Part model, mm, in its own coordinate system. Coordinates: 2 decimals unless noted, no trailing zeros. Write each loop counter-clockwise with the first axis right and the second up, starting at its lowest first coordinate (ties: lowest second). Pieces come first, ordered by that corner, then holes. Notation, with made-up numbers: M 50,-34 L 75,-34 A28 ccw 75,-4 Z; hole C 32,50.5 d3. An arc over 180 degrees is marked long. Use a Markdown table: item, result. Add a question column.
Q1. Mould opens along X. For faces 1 (the cylindrical face through (326.824, -3.131, 319.715)), 2 (the flat face through (276, -6.35, 283)), 3 (the cylindrical face through (261.402, -3.131, 293.601)) say: released by +X, released by -X, zero draft, split by the parting line, or undercut.
Q2. Slice it at C-C on y = -4.5. Count the separate pieces of the cut face and the enclosed holes in it, then the cut area to 3 significant figures.
Q3. Slice it at A-A on x = 126. Write the cut outline in (y, z).
Q4. Pin check, flat tip, straight feed: pin 1 Ø1.5 at (x, y) = (344, -5.5) entering from +Z. Stop position of the tip, or through.
Q5. Slice it at B-B on z = 308.5. Write the cut outline in (x, y), then the cut area to 3 significant figures.
Q6. Wall check: L1, parallel to Z at x = 241.5, y = -2; L2, parallel to Z at x = 363, y = -6; L3, parallel to X at y = -4.5, z = 245.5. Give the ranges that are in metal, low to high. Write a range as from..to.
from build123d import *

# Parameters (mm, degrees)
F1_DEPTH = 6.35


with BuildPart() as f1:
    # F0 (on Front) → F1 (new body)
    with BuildSketch(Plane.XZ):
        with BuildLine():
            Line((0, 420.979559), (0, 0))
            Line((0, 0), (420.979559, 0))
            ThreePointArc((420.979559, 0), (419.578436, 34.318011), (415.384391, 68.407584))
            ThreePointArc((415.384391, 68.407584), (409.893787, 72.275334), (413.730418, 77.787727))
            ThreePointArc((413.730418, 77.787727), (411.000663, 91.116653), (407.841614, 104.350407))
            ThreePointArc((407.841614, 104.350407), (402.034807, 107.724902), (405.376402, 113.550703))
            ThreePointArc((405.376402, 113.550703), (401.495342, 126.590995), (397.194916, 139.499061))
            ThreePointArc((397.194916, 139.499061), (391.116099, 142.354618), (393.937226, 148.44949))
            ThreePointArc((393.937226, 148.44949), (388.934399, 161.101903), (383.525325, 173.586043))
            ThreePointArc((383.525325, 173.586043), (377.220762, 175.90093), (379.499951, 182.218487))
            ThreePointArc((379.499951, 182.218487), (373.41343, 194.386728), (366.936875, 206.35193))
            ThreePointArc((366.936875, 206.35193), (360.454547, 208.10853), (362.174451, 214.60069))
            ThreePointArc((362.174451, 214.60069), (355.050559, 226.192152), (347.555814, 237.547355))
            ThreePointArc((347.555814, 237.547355), (340.945055, 238.732298), (342.092586, 245.349653))
            ThreePointArc((342.092586, 245.349653), (333.98554, 256.276118), (325.529643, 266.9349))
            ThreePointArc((325.529643, 266.9349), (318.840766, 267.539169), (319.407189, 274.231357))
            ThreePointArc((319.407189, 274.231357), (310.378688, 284.409668), (301.025995, 294.29091))
            ThreePointArc((301.025995, 294.29091), (294.309905, 294.309905), (294.29091, 301.025995))
            ThreePointArc((294.29091, 301.025995), (284.409668, 310.378688), (274.231357, 319.407189))
            ThreePointArc((274.231357, 319.407189), (267.539169, 318.840766), (266.9349, 325.529643))
            ThreePointArc((266.9349, 325.529643), (256.276118, 333.98554), (245.349653, 342.092586))
            ThreePointArc((245.349653, 342.092586), (238.732298, 340.945055), (237.547355, 347.555814))
            ThreePointArc((237.547355, 347.555814), (226.192152, 355.050559), (214.60069, 362.174451))
            ThreePointArc((214.60069, 362.174451), (208.10853, 360.454547), (206.35193, 366.936875))
            ThreePointArc((206.35193, 366.936875), (194.386728, 373.41343), (182.218487, 379.499951))
            ThreePointArc((182.218487, 379.499951), (175.90093, 377.220762), (173.586043, 383.525325))
            ThreePointArc((173.586043, 383.525325), (161.101903, 388.934399), (148.44949, 393.937226))
            ThreePointArc((148.44949, 393.937226), (142.354618, 391.116099), (139.499061, 397.194916))
            ThreePointArc((139.499061, 397.194916), (126.590995, 401.495342), (113.550703, 405.376402))
            ThreePointArc((113.550703, 405.376402), (107.724902, 402.034807), (104.350407, 407.841614))
            ThreePointArc((104.350407, 407.841614), (91.116653, 411.000663), (77.787727, 413.730418))
            ThreePointArc((77.787727, 413.730418), (72.275334, 409.893787), (68.407584, 415.384391))
            ThreePointArc((68.407584, 415.384391), (34.318011, 419.578436), (0, 420.979559))
        make_face()
        with BuildLine():
            Line((385.650199, 76.2), (38.1, 76.2))
            Line((38.1, 76.2), (38.1, 391.255551))
            ThreePointArc((38.1, 391.255551), (264.019048, 291.249821), (385.650199, 76.2))
        make_face(mode=Mode.SUBTRACT)
        with BuildLine():
            Line((0, 457.2), (0, 420.979559))
            ThreePointArc((0, 420.979559), (34.318011, 419.578436), (68.407584, 415.384391))
            ThreePointArc((68.407584, 415.384391), (73.503993, 419.329466), (77.864833, 414.583934))
            ThreePointArc((77.864833, 414.583934), (77.845518, 414.155438), (77.787727, 413.730418))
            ThreePointArc((77.787727, 413.730418), (91.116653, 411.000663), (104.350407, 407.841614))
            ThreePointArc((104.350407, 407.841614), (109.565802, 411.358524), (113.720028, 406.635029))
            ThreePointArc((113.720028, 406.635029), (113.677507, 406.000046), (113.550703, 405.376402))
            ThreePointArc((113.550703, 405.376402), (126.590995, 401.495342), (139.499061, 397.194916))
            ThreePointArc((139.499061, 397.194916), (144.797221, 400.283853), (148.745989, 395.591385))
            ThreePointArc((148.745989, 395.591385), (148.671278, 394.751125), (148.44949, 393.937226))
            ThreePointArc((148.44949, 393.937226), (161.101903, 388.934399), (173.586043, 383.525325))
            ThreePointArc((173.586043, 383.525325), (178.931289, 386.189559), (182.67615, 381.537053))
            ThreePointArc((182.67615, 381.537053), (182.560325, 380.493113), (182.218487, 379.499951))
            ThreePointArc((182.218487, 379.499951), (194.386728, 373.41343), (206.35193, 366.936875))
            ThreePointArc((206.35193, 366.936875), (211.70939, 369.182682), (215.25228, 364.578993))
            ThreePointArc((215.25228, 364.578993), (215.086497, 363.333362), (214.60069, 362.174451))
            ThreePointArc((214.60069, 362.174451), (226.192152, 355.050559), (237.547355, 347.555814))
            ThreePointArc((237.547355, 347.555814), (242.883215, 349.392376), (246.226455, 344.846267))
            ThreePointArc((246.226455, 344.846267), (246.001964, 343.401315), (245.349653, 342.092586))
            ThreePointArc((245.349653, 342.092586), (256.276118, 333.98554), (266.9349, 325.529643))
            ThreePointArc((266.9349, 325.529643), (272.216652, 326.968927), (275.362945, 322.489052))
            ThreePointArc((275.362945, 322.489052), (275.071106, 320.847531), (274.231357, 319.407189))
            ThreePointArc((274.231357, 319.407189), (284.409668, 310.378688), (294.29091, 301.025995))
            ThreePointArc((294.29091, 301.025995), (299.48758, 302.082614), (302.440001, 297.677501))
            ThreePointArc((302.440001, 297.677501), (302.072305, 295.842534), (301.025995, 294.29091))
            ThreePointArc((301.025995, 294.29091), (310.378688, 284.409668), (319.407189, 274.231357))
            ThreePointArc((319.407189, 274.231357), (324.489556, 274.922411), (327.251552, 270.600445))
            ThreePointArc((327.251552, 270.600445), (326.799633, 268.575526), (325.529643, 266.9349))
            ThreePointArc((325.529643, 266.9349), (333.98554, 256.276118), (342.092586, 245.349653))
            ThreePointArc((342.092586, 245.349653), (347.033388, 245.694547), (349.608767, 241.463955))
            ThreePointArc((349.608767, 241.463955), (349.064419, 239.252939), (347.555814, 237.547355))
            ThreePointArc((347.555814, 237.547355), (355.050559, 226.192152), (362.174451, 214.60069))
            ThreePointArc((362.174451, 214.60069), (366.948569, 214.620944), (369.341493, 210.48978))
            ThreePointArc((369.341493, 210.48978), (368.696688, 208.096874), (366.936875, 206.35193))
            ThreePointArc((366.936875, 206.35193), (373.41343, 194.386728), (379.499951, 182.218487))
            ThreePointArc((379.499951, 182.218487), (384.084572, 181.937522), (386.299553, 177.91365))
            ThreePointArc((386.299553, 177.91365), (385.546451, 175.34341), (383.525325, 173.586043))
            ThreePointArc((383.525325, 173.586043), (388.934399, 161.101903), (393.937226, 148.44949))
            ThreePointArc((393.937226, 148.44949), (398.311999, 147.892411), (400.353885, 143.983489))
            ThreePointArc((400.353885, 143.983489), (399.484856, 141.240809), (397.194916, 139.499061))
            ThreePointArc((397.194916, 139.499061), (401.495342, 126.590995), (405.376402, 113.550703))
            ThreePointArc((405.376402, 113.550703), (409.523557, 112.744057), (411.397529, 108.957528))
            ThreePointArc((411.397529, 108.957528), (410.405159, 106.047627), (407.841614, 104.350407))
            ThreePointArc((407.841614, 104.350407), (411.000663, 91.116653), (413.730418, 77.787727))
            ThreePointArc((413.730418, 77.787727), (417.63488, 76.759263), (419.346434, 73.102333))
            ThreePointArc((419.346434, 73.102333), (418.223548, 70.030751), (415.384391, 68.407584))
            ThreePointArc((415.384391, 68.407584), (419.578436, 34.318011), (420.979559, 0))
            Line((420.979559, 0), (457.2, 0))
            ThreePointArc((457.2, 0), (323.28922, 323.28922), (0, 457.2))
        make_face()
    extrude(amount=F1_DEPTH)


solid = f1.part
Recorded:
| question | item | result |
|---|---|---|
| 1 | face 1 | released by +X |
| 1 | face 2 | zero draft |
| 1 | face 3 | undercut |
| 2 | separate pieces | 1 |
| 2 | enclosed holes | 16 |
| 2 | area | 83,600 mm² |
| 3 | outline | M -6.35,0 L 0,0 L 0,76.2 L -6.35,76.2 Z; M -6.35,372.37 L 0,372.37 L 0,439.49 L -6.35,439.49 Z |
| 4 | pin 1 | z = 302.01 |
| 5 | outline | M 0,-6.35 L 38.1,-6.35 L 38.1,0 L 0,0 Z; M 243.64,-6.35 L 337.43,-6.35 L 337.43,0 L 243.64,0 Z |
| 5 | area | 838 mm² |
| 6 | L1 | 0..76.2, 310.18..340.08, 349.61..388.21 |
| 6 | L2 | 0..76.2, 150.88..206, 214.98..277.96 |
| 6 | L3 | 0..38.1, 307.02..342.32, 347.37..385.7 |
